from build123d import *

# Parameters (mm, degrees)
BOSS_EXTRUDE1_DEPTH = 5
FILLET1_R           = 5
SKETCH2_W           = 5
SKETCH2_H           = 115
SKETCH2_H_2         = 5
BOSS_EXTRUDE2_DEPTH = 70
SKETCH2_3_W         = 5
SKETCH2_3_H         = 105
SKETCH2_3_H_2       = 5
BOSS_EXTRUDE3_DEPTH = 50
SKETCH3_R           = 5
BOSS_EXTRUDE4_DEPTH = 70
CUT_EXTRUDE1_REACH  = 168.602
SKETCH4_W           = 7.5
SKETCH4_H           = 5
SKETCH5_R           = 2.875
SKETCH5_R_2         = 3.75
CUT_EXTRUDE2_DEPTH  = 5
SKETCH6_R           = 1.5
CUT_EXTRUDE3_DEPTH  = 5
SKETCH8_R           = 5
SKETCH8_R_2         = 2.15
BOSS_EXTRUDE5_DEPTH = 5


with BuildPart() as part:
    # Sketch1 → Boss-Extrude1 (new body)
    with BuildSketch(Plane(origin=(0, 0, 0), x_dir=(1, 0, 0), z_dir=(0, 1, 0))):
        with BuildLine():
            Line((-115, -62.5), (115, -62.5))
            ThreePointArc((115, -62.5), (122.071067812, -59.571067812), (125, -52.5))
            Line((125, -52.5), (125, 52.5))
            ThreePointArc((125, 52.5), (122.071067812, 59.571067812), (115, 62.5))
            Line((115, 62.5), (-115, 62.5))
            ThreePointArc((-115, 62.5), (-122.071067812, 59.571067812), (-125, 52.5))
            Line((-125, 52.5), (-125, -52.5))
            ThreePointArc((-125, -52.5), (-122.071067812, -59.571067812), (-115, -62.5))
        make_face()
    extrude(amount=BOSS_EXTRUDE1_DEPTH)

    # Fillet1
    fillet1_edges = [part.edges().sort_by_distance(p)[0] for p in [
        (0, 0, 62.5),
        (122.071067812, 0, 59.571067812),
        (125, 0, 0),
        (122.071067812, 0, -59.571067812),
        (0, 0, -62.5),
        (-122.071067812, 0, -59.571067812),
        (-125, 0, 0),
        (-122.071067812, 0, 59.571067812),
    ]]
    fillet(fillet1_edges, radius=FILLET1_R - 0.0001)  # a hair under: the kernel refuses the full size

    # Sketch2 → Boss-Extrude2 (add)
    with BuildSketch(Plane(origin=(0, 5, 0), x_dir=(1, 0, 0), z_dir=(0, 1, 0))):
        with Locations((12.5, 0)):
            Rectangle(SKETCH2_W, SKETCH2_H)
        with Locations((12.5, -60)):
            Rectangle(SKETCH2_W, SKETCH2_H_2)
        with BuildLine():
            Line((10, -62.5), (10, -57.5))
            Line((10, -57.5), (-115, -57.5))
            ThreePointArc((-115, -57.5), (-118.535533906, -56.035533906), (-120, -52.5))
            Line((-120, -52.5), (-120, 52.5))
            ThreePointArc((-120, 52.5), (-118.535533906, 56.035533906), (-115, 57.5))
            Line((-115, 57.5), (10, 57.5))
            Line((10, 57.5), (10, 62.5))
            Line((10, 62.5), (-115, 62.5))
            ThreePointArc((-115, 62.5), (-122.071067812, 59.571067812), (-125, 52.5))
            Line((-125, 52.5), (-125, -52.5))
            ThreePointArc((-125, -52.5), (-122.071067812, -59.571067812), (-115, -62.5))
            Line((-115, -62.5), (10, -62.5))
        make_face()
        with Locations((12.5, 60)):
            Rectangle(SKETCH2_W, SKETCH2_H_2)
    extrude(amount=BOSS_EXTRUDE2_DEPTH)

    # Sketch2<3> → Boss-Extrude3 (add)
    with BuildSketch(Plane(origin=(0, 5, 0), x_dir=(1, 0, 0), z_dir=(0, 1, 0))):
        with Locations((22.5, 0)):
            Rectangle(SKETCH2_3_W, SKETCH2_3_H)
        with BuildLine():
            Line((25, -52.5), (25, -57.5))
            Line((25, -57.5), (115, -57.5))
            ThreePointArc((115, -57.5), (118.535533906, -56.035533906), (120, -52.5))
            Line((120, -52.5), (120, 52.5))
            ThreePointArc((120, 52.5), (118.535533906, 56.035533906), (115, 57.5))
            Line((115, 57.5), (25, 57.5))
            Line((25, 57.5), (25, 52.5))
            Line((25, 52.5), (115, 52.5))
            Line((115, 52.5), (115, -52.5))
            Line((115, -52.5), (25, -52.5))
        make_face()
        with Locations((22.5, 55)):
            Rectangle(SKETCH2_3_W, SKETCH2_3_H_2)
        with Locations((22.5, -55)):
            Rectangle(SKETCH2_3_W, SKETCH2_3_H_2)
    extrude(amount=BOSS_EXTRUDE3_DEPTH)

    # Sketch3 → Boss-Extrude4 (add)
    with BuildSketch(Plane(origin=(0, 75, 0), x_dir=(1, 0, 0), z_dir=(0, 1, 0))):
        with Locations((-118.535533906, 56.035533906)):
            Circle(SKETCH3_R)
        with Locations((10, 57.5)):
            Circle(SKETCH3_R)
        with Locations((10, -57.5)):
            Circle(SKETCH3_R)
        with Locations((-118.535533906, -56.035533906)):
            Circle(SKETCH3_R)
    extrude(amount=-BOSS_EXTRUDE4_DEPTH)

    # Cut-Extrude1: up to this face of the body (flat: up to its plane)
    cut_extrude1_end = Plane(part.part.faces().sort_by_distance((25, 30, 0))[0])
    # Sketch4 → Cut-Extrude1 (cut, up to the picked face)
    with BuildSketch(Plane.ZY.offset(-10), mode=Mode.PRIVATE) as cut_extrude1_sk1:
        with Locations((0, 7.5)):
            Rectangle(SKETCH4_W, SKETCH4_H)
    cut_extrude1_tool1 = split(extrude(cut_extrude1_sk1.sketch, amount=-CUT_EXTRUDE1_REACH, mode=Mode.PRIVATE), bisect_by=cut_extrude1_end, keep=Keep.BOTH, mode=Mode.PRIVATE)
    add(cut_extrude1_tool1.solids().sort_by(Axis((10, 7.5, 0), (1, 0, 0)))[0], mode=Mode.SUBTRACT)

    # Sketch5 → Cut-Extrude2 (cut)
    with BuildSketch(Plane.XY.offset(-57.5)):
        with Locations((-96, 13)):
            Circle(SKETCH5_R)
        with Locations((-10, 60)):
            Circle(SKETCH5_R_2)
    extrude(amount=-CUT_EXTRUDE2_DEPTH, mode=Mode.SUBTRACT)

    # Sketch6 → Cut-Extrude3 (cut)
    with BuildSketch(Plane.XY.offset(62.5)):
        with Locations((-105, 15)):
            Circle(SKETCH6_R)
        with Locations((-98, 15)):
            Circle(SKETCH6_R)
        with Locations((-91, 15)):
            Circle(SKETCH6_R)
    extrude(amount=-CUT_EXTRUDE3_DEPTH, mode=Mode.SUBTRACT)

    # Sketch8 → Boss-Extrude5 (add)
    # profile 1 of 4: a face of its own
    with BuildSketch(Plane(origin=(0, 5, 0), x_dir=(1, 0, 0), z_dir=(0, 1, 0))):
        with Locations(Location((-100, -37.5, 0), (0, 0, 90))):
            Circle(SKETCH8_R)
        with Locations(Location((-100, -37.5, 0), (0, 0, 270))):
            Circle(SKETCH8_R_2, mode=Mode.SUBTRACT)
    # profile 2 of 4: a face of its own
    with BuildSketch(Plane(origin=(0, 5, 0), x_dir=(1, 0, 0), z_dir=(0, 1, 0))):
        with Locations(Location((-58, -37.5, 0), (0, 0, 90))):
            Circle(SKETCH8_R)
        with Locations(Location((-58, -37.5, 0), (0, 0, 270))):
            Circle(SKETCH8_R_2, mode=Mode.SUBTRACT)
    # profile 3 of 4: a face of its own
    with BuildSketch(Plane(origin=(0, 5, 0), x_dir=(1, 0, 0), z_dir=(0, 1, 0))):
        with Locations(Location((-58, 22.5, 0), (0, 0, 90))):
            Circle(SKETCH8_R)
        with Locations(Location((-58, 22.5, 0), (0, 0, 270))):
            Circle(SKETCH8_R_2, mode=Mode.SUBTRACT)
    # profile 4 of 4: a face of its own
    with BuildSketch(Plane(origin=(0, 5, 0), x_dir=(1, 0, 0), z_dir=(0, 1, 0))):
        with Locations(Location((-100, 22.5, 0), (0, 0, 90))):
            Circle(SKETCH8_R)
        with Locations(Location((-100, 22.5, 0), (0, 0, 270))):
            Circle(SKETCH8_R_2, mode=Mode.SUBTRACT)
    extrude(amount=BOSS_EXTRUDE5_DEPTH)


solid = part.part
Build history of the part. All positions in model axes, mm. A direction names the side the tool comes from. Give positions to 0.01 mm unless a question says otherwise; leave off trailing zeros. Loops run counter-clockwise (first coordinate to the right, second up) from the corner with the lowest first, then second, coordinate; pieces in that order, holes last. Notation, with made-up numbers: (51.5, -19.5) - (108.5, -19.5) arc R18 cw to (108.5, 14.5) - close; hole circle Ø2 at (52.5, -28). An arc over 180 degrees is marked (long way). Write item = value, one per line. Start each with the question number.
1) Drop flat-ended pins along their axis: pin 1 Ø10 at (y, z) = (26, -15.5) entering from +X; pin 2 Ø4 at (x, z) = (-58, -22.5) entering from +Y; pin 3 Ø11 at (x, z) = (-59, 38.5) entering from +Y. Give the stop position or say it passes through.
2) Probe probe 1 along X at (y, z) = (27.5, -28.5); probe 2 along Z at (x, y) = (-83, 59); probe 3 along Z at (x, y) = (27.5, 33). List the from-to ranges inside material, lowest first. Write a range as from..to.
3) Band-saw the part on A-A on y = 24. Give the cut face in (x, z).
4) Band-saw the part on B-B on x = -10. Give the cut face in (y, z).
5) Tool access for faces 1 (the cylindrical face through (6.43, 40.49, -54)), 2 (the flat face through (68, 30, -57.5)), 3 (the flat face through (20, 30, -1)): list every direction of +Z, -Z, +X, -X, +Y, -Y with a clear straight run to the whole face (end or side of a thin tool).
6) Band-saw the part on D-D on x = -46. Give the cut face in (y, z).
7) Pull direction Y, two halves, no side cores. Call faces 4 (the flat face through (71, 30, 52.5)), 5 (the flat face through (12, 7, 3.75)), 6 (the cylindrical face through (1.61, 1.5, 61.07)), 7 (the cylindrical face through (-93.344, 11.899, -59.965)): +Y half, -Y half, draft (parallel to the pull), parting line (faces both ways), or undercut.
Final values:
q1.pin_1 = 120
q1.pin_2 = 5
q1.pin_3 = 10
q2.probe_1 = -125..-120, 10..15, 20..25, 115..120
q2.probe_2 = -62.5..-57.5, 57.5..62.5
q2.probe_3 = -57.5..-52.5, 52.5..57.5
q3.outline = (-125, -52.5) arc R10 ccw to (-115, -62.5) - (15, -62.5) - (15, 62.5) - (-115, 62.5) arc R10 ccw to (-125, 52.5) - close; (20, -57.5) - (115, -57.5) arc R5 ccw to (120, -52.5) - (120, 52.5) arc R5 ccw to (115, 57.5) - (20, 57.5) - close; hole (-120, -51.25) arc R5 cw to (-113.75, -57.5) - (5, -57.5) arc R5 cw to (10, -52.5) - (10, 52.5) arc R5 cw to (5, 57.5) - (-113.75, 57.5) arc R5 cw to (-120, 51.25) - close; hole (25, -52.5) - (115, -52.5) - (115, 52.5) - (25, 52.5) - close
q4.outline = (0, -57.5) arc R5 ccw to (5, -62.5) - (56.25, -62.5) - (56.25, -57.5) - (5, -57.5) - (5, 57.5) - (75, 57.5) - (75, 62.5) - (5, 62.5) arc R5 ccw to (0, 57.5) - close; (63.75, -62.5) - (75, -62.5) - (75, -57.5) - (63.75, -57.5) - close
q5.face_1 = +Y
q5.face_2 = -Z, +X, +Y
q5.face_3 = +Z, -Z, +Y
q6.outline = (0, -57.5) arc R5 ccw to (5, -62.5) - (75, -62.5) - (75, -57.5) - (5, -57.5) - (5, 57.5) - (75, 57.5) - (75, 62.5) - (5, 62.5) arc R5 ccw to (0, 57.5) - close
q7.face_4 = draft
q7.face_5 = undercut
q7.face_6 = -Y half
q7.face_7 = undercut
